Part model, mm, in its own coordinate system. Face numbers are marked on the shaded views. A direction names the side the tool comes from. Round coordinates to 2 decimals unless told otherwise and drop trailing zeros. Loops run counter-clockwise (first coordinate to the right, second up) from the corner with the lowest first, then second, coordinate; pieces in that order, holes last. Notation, with made-up numbers: (80, -19.5) - (126, -19.5) arc R11 cw to (126, -15.5) - close; hole circle Ø8 at (58, -2). An arc over 180 degrees is marked (long way). Put each result on its own line as item: value.
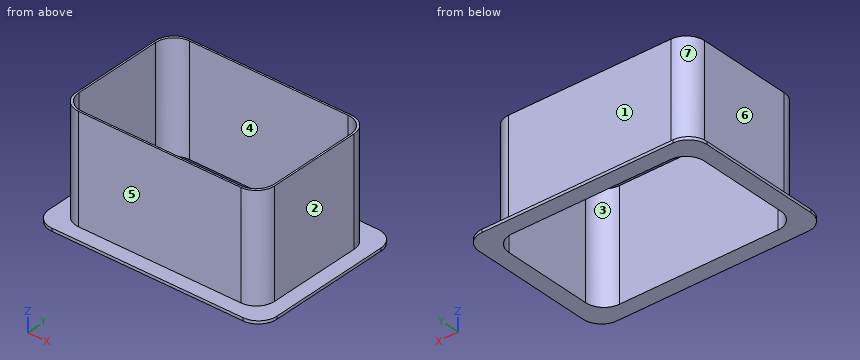
from build123d import *

# Parameters (mm, degrees)
PAD_DEPTH    = 75
PAD005_DEPTH = 2
POCKET_DEPTH = 75.001


with BuildPart() as part:
    # Sketch → Pad (new body)
    with BuildSketch(Plane.XY):
        with BuildLine():
            Line((55.9, 45), (-55.9, 45))
            ThreePointArc((-55.9, 45), (-64.809545, 41.309545), (-68.5, 32.4))
            Line((-68.5, 32.4), (-68.5, -32.4))
            ThreePointArc((-68.5, -32.4), (-64.809545, -41.309545), (-55.9, -45))
            Line((-55.9, -45), (55.9, -45))
            ThreePointArc((55.9, -45), (64.809545, -41.309545), (68.5, -32.4))
            Line((68.5, -32.4), (68.5, 32.4))
            ThreePointArc((68.5, 32.4), (64.809545, 41.309545), (55.9, 45))
        make_face()
    extrude(amount=PAD_DEPTH)

    # Sketch006 → Pad005 (join)
    with BuildSketch(Plane.XY):
        with BuildLine():
            Line((-65.9, 55), (65.9, 55))
            ThreePointArc((78.5, 42.4), (74.809545, 51.309545), (65.9, 55))
            Line((78.5, 42.4), (78.5, -42.4))
            ThreePointArc((65.9, -55), (74.809545, -51.309545), (78.5, -42.4))
            Line((65.9, -55), (-65.9, -55))
            ThreePointArc((-78.5, -42.4), (-74.809545, -51.309545), (-65.9, -55))
            Line((-78.5, -42.4), (-78.5, 42.4))
            ThreePointArc((-65.9, 55), (-74.809545, 51.309545), (-78.5, 42.4))
        make_face()
    extrude(amount=PAD005_DEPTH)

    # Sketch007 → Pocket (cut, through all)
    with BuildSketch(Plane.XY):
        with BuildLine():
            Line((-54.7, 43.8), (54.7, 43.8))
            ThreePointArc((67.3, 31.2), (63.609545, 40.109545), (54.7, 43.8))
            Line((67.3, 31.2), (67.3, -31.2))
            ThreePointArc((54.7, -43.8), (63.609545, -40.109545), (67.3, -31.2))
            Line((54.7, -43.8), (-54.7, -43.8))
            ThreePointArc((-67.3, -31.2), (-63.609545, -40.109545), (-54.7, -43.8))
            Line((-67.3, -31.2), (-67.3, 31.2))
            ThreePointArc((-54.7, 43.8), (-63.609545, 40.109545), (-67.3, 31.2))
        make_face()
    extrude(amount=POCKET_DEPTH, mode=Mode.SUBTRACT)


solid = part.part
1. Probe line 1 along X through (y, z) = (-16, 35.5); line 2 along Y through (x, z) = (2, 7.5); line 3 along Z through (x, y) = (71.5, 48.5). List the from-to ranges inside material, lowest first. Write a range as [from, to].
A:
line 1: x = [-68.5, -67.3], [67.3, 68.5]
line 2: y = [-45, -43.8], [43.8, 45]
line 3: z = [0, 2]
2. Two-plate mould, pull along Y, no slides. Class the marked faces 4, 5, 6 and 7: pulls with the +Y half, pulls with the -Y half, needs draft (parallel to the pull), parting line crosses it, or undercut.
A:
face 4: undercut
face 5: pulls with the -Y half
face 6: needs draft
face 7: pulls with the +Y half
3. Band-saw the part on A-A (x = -27). List the corners of the cut face in (y, z), plus the area to 3 significant figures.
A:
outline: (-55, 0) - (-43.8, 0) - (-43.8, 75) - (-45, 75) - (-45, 2) - (-55, 2) - close; (43.8, 0) - (55, 0) - (55, 2) - (45, 2) - (45, 75) - (43.8, 75) - close
area: 220 mm²
4. Band-saw the part on B-B (z = 58). List the corners of the cut face in (x, y), plus the area to 3 significant figures.
A:
outline: (-68.5, -32.4) arc R12.6 ccw to (-55.9, -45) - (55.9, -45) arc R12.6 ccw to (68.5, -32.4) - (68.5, 32.4) arc R12.6 ccw to (55.9, 45) - (-55.9, 45) arc R12.6 ccw to (-68.5, 32.4) - close; hole (-67.3, -31.2) arc R12.6 ccw to (-54.7, -43.8) - (54.7, -43.8) arc R12.6 ccw to (67.3, -31.2) - (67.3, 31.2) arc R12.6 ccw to (54.7, 43.8) - (-54.7, 43.8) arc R12.6 ccw to (-67.3, 31.2) - close
area: 539 mm²
5. Pin check, flat tips, straight feed: P1, Ø2, axis at y = -40.5, z = 30, coming from the +X side; P2, Ø1.5, axis at x = -56.5, z = 21.5, coming from the +Y side; P3, Ø1, axis at y = 8.5, z = 40, coming from the -X side. Stop position of each tip, or through.
A:
P1: stops at x = 66.31
P2: stops at y = 45
P3: stops at x = -68.5
6. Tool access for the marked faces 1, 2 and 3: list every direction of +Z, -Z, +X, -X, +Y, -Y with a clear straight run to the whole face (end or side of a thin tool).
A:
face 1: +Z, +X, -X, +Y
face 2: +Z, +X, +Y, -Y
face 3: +Z, -Z
7. Band-saw the part on C-C (y = 0). List the corners of the cut face in (x, z).
A:
outline: (-78.5, 0) - (-67.3, 0) - (-67.3, 75) - (-68.5, 75) - (-68.5, 2) - (-78.5, 2) - close; (67.3, 0) - (78.5, 0) - (78.5, 2) - (68.5, 2) - (68.5, 75) - (67.3, 75) - close
